```python
from build123d import *

# Parameters (mm, degrees)
ESQUISSE1_R                                = 11
BOSS_EXTRU_1_DEPTH                         = 5
BOSS_EXTRU_2_DEPTH                         = 5
CONG_1_R                                   = 0.5
CONG_2_R                                   = 0.5
CHAMBRAGE_POUR_VIS_T_TE_HEXAGONALE_2_COUNT = 2
CHAMBRAGE_POUR_VIS_T_TE_HEXAGONALE_2_PITCH = 14


with BuildPart() as part:
    # Esquisse1 → Boss.-Extru.1 (new body)
    with BuildSketch(Plane.XY):
        Circle(ESQUISSE1_R)
    extrude(amount=BOSS_EXTRU_1_DEPTH)

    # Esquisse2 → Boss.-Extru.2 (add)
    with BuildSketch(Plane.XY.offset(5)):
        with BuildLine():
            Line((-2.25, 10.767427734), (-2.25, -10.767427734))
            ThreePointArc((-2.25, -10.767427734), (0, -11), (2.25, -10.767427734))
            Line((2.25, -10.767427734), (2.25, 10.767427734))
            ThreePointArc((2.25, 10.767427734), (0, 11), (-2.25, 10.767427734))
        make_face()
    extrude(amount=BOSS_EXTRU_2_DEPTH)

    # Congé1
    # the kernel refuses this fillet: 0.5 mm, written as the material it takes off along each edge
    with BuildSketch(Plane(origin=(0, 0, 5), x_dir=(1, 0, 0), z_dir=(0, -1, 0))) as cong_1_piece_1_section:
        with BuildLine():
            CenterArc((11 - CONG_1_R, -CONG_1_R), CONG_1_R, 0, 90)
            Line((11 - CONG_1_R, 0), (11, 0))
            Line((11, 0), (11, -CONG_1_R))
        make_face()
    cong_1_piece_1 = revolve(axis=Axis((0, 0, 5), (0, 0, 1)), revolution_arc=84.709966663, mode=Mode.PRIVATE)
    cong_1_piece_1 = split(cong_1_piece_1, bisect_by=Plane(origin=(2.25, 6.849238197, 4.860494097), z_dir=(1, 0, 0)), keep=Keep.TOP, mode=Mode.PRIVATE)
    add(cong_1_piece_1, mode=Mode.SUBTRACT)
    with BuildSketch(Plane(origin=(0, 0, 5), x_dir=(-0.09209435598591774, 0.9957502847579502, 0), z_dir=(0.9957502847579502, 0.09209435598591774, 0))) as cong_1_piece_2_section:
        with BuildLine():
            CenterArc((11 - CONG_1_R, -CONG_1_R), CONG_1_R, 0, 90)
            Line((11 - CONG_1_R, 0), (11, 0))
            Line((11, 0), (11, -CONG_1_R))
        make_face()
    cong_1_piece_2 = revolve(axis=Axis((0, 0, 5), (0, 0, 1)), revolution_arc=169.431789296, mode=Mode.PRIVATE)
    cong_1_piece_2 = split(cong_1_piece_2, bisect_by=Plane(origin=(-2.25, 0, 4.86229808), z_dir=(-1, 0, 0)), keep=Keep.TOP, mode=Mode.PRIVATE)
    add(cong_1_piece_2, mode=Mode.SUBTRACT)
    with BuildSketch(Plane(origin=(0, 0, 5), x_dir=(0.09219737865829941, -0.9957407510836032, 0), z_dir=(-0.9957407510836032, -0.09219737865829941, 0))) as cong_1_piece_3_section:
        with BuildLine():
            CenterArc((11 - CONG_1_R, -CONG_1_R), CONG_1_R, 0, 90)
            Line((11 - CONG_1_R, 0), (11, 0))
            Line((11, 0), (11, -CONG_1_R))
        make_face()
    cong_1_piece_3 = revolve(axis=Axis((0, 0, 5), (0, 0, 1)), revolution_arc=84.709966663, mode=Mode.PRIVATE)
    cong_1_piece_3 = split(cong_1_piece_3, bisect_by=Plane(origin=(2.25, -6.849238209, 4.860494116), z_dir=(1, 0, 0)), keep=Keep.TOP, mode=Mode.PRIVATE)
    add(cong_1_piece_3, mode=Mode.SUBTRACT)

    # Congé2
    cong_2_edges = [part.edges().sort_by_distance(p)[0] for p in [
        (-2.25, 0, 10),
        (2.25, 0, 10),
    ]]
    fillet(cong_2_edges, radius=CONG_2_R)

    # Esquisse4 → Chambrage pour vis à tête hexagonale M31 (revolve, cut)
    with BuildSketch(Plane(origin=(-7, 0, 5), x_dir=(0, -1, 0), z_dir=(1, 0, 0))):
        Polygon((0, 0), (0, 5), (1.7, 5), (1.7, 2), (4.6755, 2), (4.6755, 0.025), (4.7005, 0), align=None)
    chambrage_pour_vis_t_te_hexagonale_m31 = revolve(axis=Axis((-7, 0, 11.35), (0, 0, -1)), mode=Mode.SUBTRACT)

    # Chambrage pour vis _ t_te hexagonale 2: Chambrage pour vis à tête hexagonale M31 ×2
    with Locations(*[(i * CHAMBRAGE_POUR_VIS_T_TE_HEXAGONALE_2_PITCH, 0, 0) for i in range(1, CHAMBRAGE_POUR_VIS_T_TE_HEXAGONALE_2_COUNT)]):
        add(chambrage_pour_vis_t_te_hexagonale_m31, mode=Mode.SUBTRACT)


solid = part.part
```
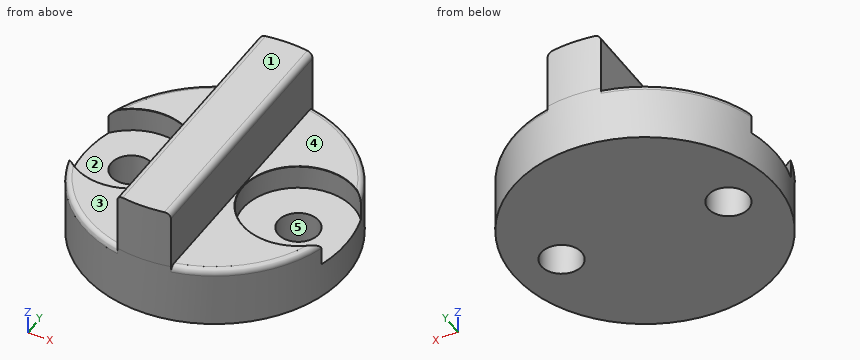
Source: CAD feature listing. Evaluate the final solid. Frame: model axes, mm. Face numbers are marked on the shaded views. A direction names the side the tool comes from. Round coordinates to 2 decimals unless told otherwise and drop trailing zeros. Loops run counter-clockwise (first coordinate to the right, second up) from the corner with the lowest first, then second, coordinate; pieces in that order, holes last. Notation, with made-up numbers: M -2.5,67.5 L 31.5,67.5 A21 ccw 31.5,90.5 Z; hole C -3,38 d9. An arc over 180 degrees is marked long. Use a Markdown table: item, result. Add a question column.
1. Contact query for flat-ended pins moving along their axis: P1, Ø6, axis at y = 5, z = 3.5, coming from the +X side; P2, Ø4.5, axis at x = 7, y = 0, coming from the -Z side; P3, Ø3, axis at x = -7, y = 0, coming from the -Z side; P4, Ø5.5, axis at y = 0.5, z = 6.5, coming from the -X side. Output: stop coordinate, or through.
2. Reachability of the marked faces 1, 2, 3, 4 and 5 from +Z, -Z, +X, -X, +Y, -Y: full face, straight path, thin tool, end or side. Return the list, or none.
3. Section query A-A on y = 0. Give the number of separate pieces and of enclosed holes in the cut face, then the cut area to 3 significant figures.
4. Section query B-B on z = 6.25. Return the cut outline in (x, y).
5. Line query: line 1 (X direction, y = 0, z = 1.25); line 2 (Z direction, x = -2.75, y = 9); line 3 (X direction, y = 6.5, z = 5.25). Output: solid intervals per line, ascending.
6. Section query C-C on z = 4. Return the cut outline in (x, y).
Reported:
| question | item | result |
|---|---|---|
| 1 | P1 | stops at x = 10.81 |
| 1 | P2 | stops at z = 0 |
| 1 | P3 | passes through |
| 1 | P4 | stops at x = -3.25 |
| 2 | face 1 | +Z, +X, -X, +Y, -Y |
| 2 | face 2 | +Z |
| 2 | face 3 | +Z, -X, +Y, -Y |
| 2 | face 4 | +Z, +X, +Y, -Y |
| 2 | face 5 | +Z, -Z |
| 3 | separate pieces | 3 |
| 3 | enclosed holes | 0 |
| 3 | area | 77.3 mm² |
| 4 | outline | M -2.25,-10.77 A11 ccw 2.25,-10.77 L 2.25,10.77 A11 ccw -2.25,10.77 Z |
| 5 | line 1 | x = -11 to -8.7, -5.3 to 5.3, 8.7 to 11 |
| 5 | line 2 | z = 0 to 5 |
| 5 | line 3 | x = -2.25 to 2.25 |
| 6 | outline | M -10.58,-3.01 A11 ccw 10.58,-3.01 A4.68 cw long 10.58,3.01 A11 ccw -10.58,3.01 A4.68 cw long Z |
